Source: CAD feature listing. Evaluate the final solid. Frame: model axes, mm. Give positions to 0.01 mm unless a question says otherwise; leave off trailing zeros. Write each loop counter-clockwise with the first axis right and the second up, starting at its lowest first coordinate (ties: lowest second). Pieces come first, ordered by that corner, then holes. Notation, with made-up numbers: (-39, -38) -> (-26, -38) arc R31 ccw to (-26, -8) -> close; hole circle Ø1 at (-9, -17.75). An arc over 180 degrees is marked (long way). Answer as a JSON object with one key per item and string values. Group by question number.
Item 1: First-contact query: pin 1 Ø2 at (x, y) = (41.5, 5) entering from -Z; pin 2 Ø2 at (y, z) = (2, 85.5) entering from +X; pin 3 Ø3 at (x, y) = (80.5, 5) entering from -Z. Flat tips, straight axial feed; report the tip coordinate or a pass-through.
Item 2: Section query A-A on x = 0. Return the cut outline in (y, z).
Item 3: Section query B-B on z = 0. Return the cut outline in (x, y).
Item 4: Pull-direction query (Z, two-part tool) for faces 1 (the face through (-38.4, 0, -70.5)), 2 (the face through (-58.72, 3.4, 64.77)), 3 (the face through (31.54, 3.3, 100.15)); classes: pulls with the +Z half, pulls with the -Z half, needs draft (parallel to the pull), parting line crosses it, or undercut.
Item 5: Ray query, probe 1 along X at (y, z) = (1.75, -45.5); probe 2 along Z at (x, y) = (-62, 6.5); probe 3 along X at (y, z) = (3.5, -2.5). Return the intervals inside material, ascending. Write a range as from..to.
Item 6: Section query D-D on z = 67.5. Return the cut outline in (x, y), plus the area to 3 significant figures.
from build123d import *

# Parameters (mm, degrees)
SKETCH1_R           = 105
SKETCH1_R_2         = 80
BOSS_EXTRUDE1_DEPTH = 6.7
SKETCH2_W           = 6.7
SKETCH2_H           = 20
CUT_EXTRUDE3_DEPTH  = 6.7


with BuildPart() as part:
    # Sketch1 → Boss-Extrude1 (new body)
    with BuildSketch(Plane(origin=(0, 0, 0), x_dir=(1, 0, 0), z_dir=(0, 1, 0))):
        with Locations(Location((0, 0, 0), (0, 0, 270))):
            Circle(SKETCH1_R)
        with Locations(Location((0, 0, 0), (0, 0, 270))):
            Circle(SKETCH1_R_2, mode=Mode.SUBTRACT)
    extrude(amount=BOSS_EXTRUDE1_DEPTH)

    # Sketch2 → Cut-Extrude3 (cut)
    with BuildSketch(Plane(origin=(0, 6.7, 0), x_dir=(1, 0, 0), z_dir=(0, 1, 0))):
        Polygon((80.59741336, 50.401185103), (63.276905284, 40.401185103), (66.626905284, 34.598814897), (83.94741336, 44.598814897), align=None)
        Polygon((63.631071805, -70.620883604), (50.775319611, -55.299994741), (45.642821842, -59.606671726), (58.498574036, -74.927560589), align=None)
        Polygon((94.138457931, -13.197470906), (74.442302871, -9.724507352), (73.278860081, -16.322719298), (92.975015141, -19.795682851), align=None)
        with Locations((0, -85)):
            Rectangle(SKETCH2_W, SKETCH2_H)
        Polygon((-58.498574036, -74.927560589), (-45.642821842, -59.606671726), (-50.775319611, -55.299994741), (-63.631071805, -70.620883604), align=None)
        Polygon((-92.975015141, -19.795682851), (-73.278860081, -16.322719298), (-74.442302871, -9.724507352), (-94.138457931, -13.197470906), align=None)
        Polygon((-83.94741336, 44.598814897), (-66.626905284, 34.598814897), (-63.276905284, 40.401185103), (-80.59741336, 50.401185103), align=None)
    extrude(amount=-CUT_EXTRUDE3_DEPTH, mode=Mode.SUBTRACT)


solid = part.part
Worked answers:
{
 "1": {"pin 1": "z = -96.87", "pin 2": "x = 62.33", "pin 3": "z = -69.17"},
 "2": {"outline": "(0, -105) -> (6.7, -105) -> (6.7, -80) -> (0, -80) -> close; (0, 95) -> (6.7, 95) -> (6.7, 105) -> (0, 105) -> close"},
 "3": {"outline": "(-105, 0) -> (-80, 0) -> (-80, 6.7) -> (-105, 6.7) -> close; (80, 0) -> (105, 0) -> (105, 6.7) -> (80, 6.7) -> close"},
 "4": {"face 1": "needs draft", "face 2": "undercut", "face 3": "parting line crosses it"},
 "5": {"probe 1": "-94.63..-83.43, -72.11..-65.8, 65.8..72.11, 83.43..94.63", "probe 2": "-84.74..-50.56, 50.56..68.68, 71.99..84.74", "probe 3": "-104.97..-79.96, 79.96..104.97"},
 "6": {"outline": "(-80.43, 0) -> (-61.01, 0) -> (-61.01, 6.7) -> (-80.43, 6.7) -> close; (-52.27, 0) -> (-42.94, 0) -> (-42.94, 6.7) -> (-52.27, 6.7) -> close; (42.94, 0) -> (52.27, 0) -> (52.27, 6.7) -> (42.94, 6.7) -> close; (61.01, 0) -> (80.43, 0) -> (80.43, 6.7) -> (61.01, 6.7) -> close", "area": "385 mm^2"}
}
